Source: CAD feature listing. Evaluate the final solid. Frame: model axes, mm. Face numbers are marked on the shaded views. A direction names the side the tool comes from. Give positions to 0.01 mm unless a question says otherwise; leave off trailing zeros. Write each loop counter-clockwise with the first axis right and the second up, starting at its lowest first coordinate (ties: lowest second). Pieces come first, ordered by that corner, then holes. Notation, with made-up numbers: M -31,51 L -13,51 A33 ccw -13,87 Z; hole C 10.5,41 d8. An arc over 180 degrees is marked long. Return JSON: item names as keys, results as strings.
```python
from build123d import *

# Parameters (mm, degrees)
SKETCH_1_W          = 77
SKETCH_1_H          = 145
EXTRUDE_1_DEPTH     = 1.5
EXTRUDE_2_DEPTH     = 40
SKETCH_3_W          = 74
SKETCH_3_H          = 1.5
EXTRUDE_3_DEPTH     = 10
SKETCH_4_W          = 3
SKETCH_4_H          = 22
CUT_EXTRUDE_1_DEPTH = 100


with BuildPart() as part:
    # Эскиз1 → Бобышка-Вытянуть1 (new body)
    with BuildSketch(Plane.XY):
        with Locations((38.5, 72.5)):
            Rectangle(SKETCH_1_W, SKETCH_1_H)
    extrude(amount=EXTRUDE_1_DEPTH)

    # Эскиз2 → Бобышка-Вытянуть2 (add)
    with BuildSketch(Plane.XY.offset(1.5)):
        Polygon((1.5, 145), (1.5, 1.5), (75.5, 1.5), (75.5, 145), (77, 145), (77, 0), (0, 0), (0, 145), align=None)
    extrude(amount=EXTRUDE_2_DEPTH)

    # Эскиз3 → Бобышка-Вытянуть3 (add)
    with BuildSketch(Plane.XY.offset(1.5)):
        with Locations((38.5, 144.25)):
            Rectangle(SKETCH_3_W, SKETCH_3_H)
    extrude(amount=EXTRUDE_3_DEPTH)

    # Эскиз4 → Вырез-Вытянуть1 (cut)
    with BuildSketch(Plane(origin=(77, 0, 0), x_dir=(0, 0, -1), z_dir=(1, 0, 0))):
        with Locations((-3, 114)):
            Rectangle(SKETCH_4_W, SKETCH_4_H)
        with Locations((-3, 31)):
            Rectangle(SKETCH_4_W, SKETCH_4_H)
    extrude(amount=-CUT_EXTRUDE_1_DEPTH, mode=Mode.SUBTRACT)


solid = part.part
```
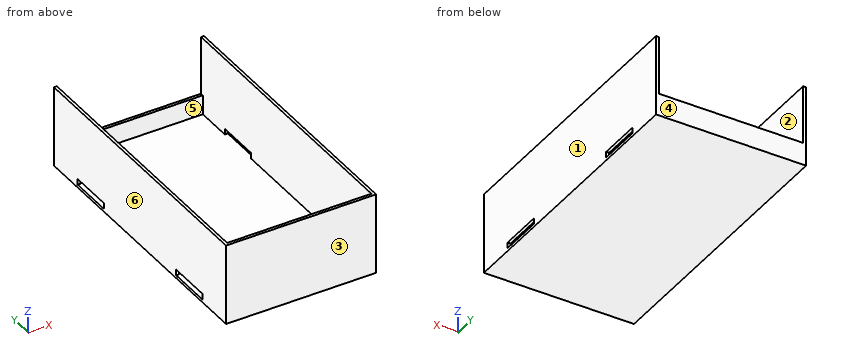
1) Cut plane C-C, the plane y = 77. Return the cut outline in (x, z).
Numbers:
{"outline": "M 0,0 L 77,0 L 77,41.5 L 75.5,41.5 L 75.5,1.5 L 1.5,1.5 L 1.5,41.5 L 0,41.5 Z"}
2) Draft query along Y for the marked faces 1, 2, 3 and 4. Return one class per face: released by +Y, released by -Y, zero draft, split by the parting line, or undercut.
Numbers:
{"face 1": "zero draft", "face 2": "undercut", "face 3": "released by -Y", "face 4": "released by +Y"}
3) Set-up query: the marked faces 5 and 6. Return all of +Z, -Z, +X, -X, +Y, -Y with unobstructed straight access to the full face (end or side cutting, diameter ignored); none if empty.
Numbers:
{"face 5": "+Z", "face 6": "+Z, -Z, -X, +Y, -Y"}
4) Cut plane A-A, the plane y = 29.5. Return the cut outline in (x, z).
Numbers:
{"outline": "M 0,0 L 77,0 L 77,1.5 L 0,1.5 Z; M 0,4.5 L 1.5,4.5 L 1.5,41.5 L 0,41.5 Z; M 75.5,4.5 L 77,4.5 L 77,41.5 L 75.5,41.5 Z"}
5) Contact query for a flat-ended pin moving along its axis: pin 1 Ø1 at (x, y) = (52, 101.5) entering from +Z. Output: stop coordinate, or through.
Numbers:
{"pin 1": "stops at z = 1.5"}
6) Cut plane B-B, the plane z = 13. Return the cut outline in (x, y), then the cut area to 3 significant figures.
Numbers:
{"outline": "M 0,0 L 77,0 L 77,145 L 75.5,145 L 75.5,1.5 L 1.5,1.5 L 1.5,145 L 0,145 Z", "area": "546 mm²"}
7) Line query: line 1 (X direction, y = 33.5, z = 22.5); line 2 (Y direction, x = 59.5, z = 6); line 3 (Z direction, x = 66.5, y = 99). Output: solid intervals per line, ascending. Write a range as [from, to].
Numbers:
{"line 1": "x = [0, 1.5], [75.5, 77]", "line 2": "y = [0, 1.5], [143.5, 145]", "line 3": "z = [0, 1.5]"}
